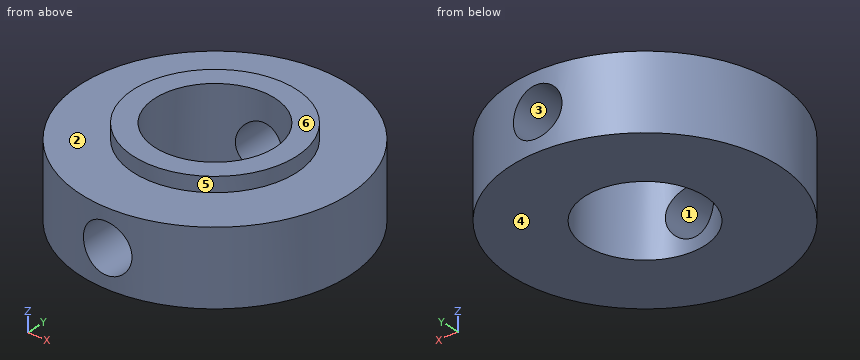
from build123d import *

# Parameters (mm, degrees)
ESQUISSE1_R                  = 9.05
ESQUISSE1_R_2                = 4.05
BOSS_EXTRU_1_DEPTH           = 5
ENL_V_MAT_EXTRU_1_DEPTH      = 14.740633173
ENL_V_MAT_EXTRU_1_DEPTH_BACK = 14.740633173
ESQUISSE2_R                  = 1.65
ESQUISSE3_R                  = 5.5
ESQUISSE3_R_2                = 4.05
BOSS_EXTRU_2_DEPTH           = 1


with BuildPart() as part:
    # Esquisse1 → Boss.-Extru.1 (new body)
    with BuildSketch(Plane.XY):
        Circle(ESQUISSE1_R)
        Circle(ESQUISSE1_R_2, mode=Mode.SUBTRACT)
    extrude(amount=BOSS_EXTRU_1_DEPTH)

    # Esquisse2 → Enlèv. mat.-Extru.1 (cut, two sides: drawn at the far end of the back side and taken through both)
    with BuildSketch(Plane(origin=(0, 0, 0), x_dir=(1, 0, 0), z_dir=(0, 1, 0)).offset(-ENL_V_MAT_EXTRU_1_DEPTH_BACK)):
        with Locations(Location((0, -2.5, 0), (0, 0, 270))):
            Circle(ESQUISSE2_R)
    extrude(amount=ENL_V_MAT_EXTRU_1_DEPTH + ENL_V_MAT_EXTRU_1_DEPTH_BACK, mode=Mode.SUBTRACT)

    # Esquisse3 → Boss.-Extru.2 (add)
    with BuildSketch(Plane.XY.offset(5)):
        Circle(ESQUISSE3_R)
        Circle(ESQUISSE3_R_2, mode=Mode.SUBTRACT)
    extrude(amount=BOSS_EXTRU_2_DEPTH)


solid = part.part
The model under review builds one solid part; all positions refer to its coordinate system, in mm. Face numbers are marked on the shaded views. A direction names the side the tool comes from. Give positions to 0.01 mm unless a question says otherwise; leave off trailing zeros. Loops run counter-clockwise (first coordinate to the right, second up) from the corner with the lowest first, then second, coordinate; pieces in that order, holes last. Notation, with made-up numbers: (74, 43.5) -> (78, 43.5) arc R28 cw to (78, 82.5) -> close; hole circle Ø10 at (-24.75, -30). An arc over 180 degrees is marked (long way). Answer as a JSON object with one key per item and string values. Group by question number.
Q1. Tool access review of the marked faces 1 and 2: name each direction out of +Z, -Z, +X, -X, +Y, -Y from which nothing blocks a thin tool from reaching the whole face with its end or side.
Q2. Take a section at B-B (x = 0). Write out the cut boundary in (y, z), plus the area to 3 significant figures.
Q3. Take a section at D-D (z = 2.5). Write out the cut boundary in (x, y).
Q4. Draft analysis for pull direction Z (two halves, no side actions). For the marked faces 3, 4, 5 and 6, state which applies: pulls with the +Z half, pulls with the -Z half, needs draft (parallel to the pull), parting line crosses it, or undercut.
Q5. Wall thickness on line 1 along Z through (x, y) = (0, -6.35); line 2 along Z through (x, y) = (-6.75, -2); line 3 along X through (y, z) = (-6.15, 2.5): over which ranges is each line inside the solid? List them lowest first.
Q6. Take a section at A-A (y = 0). Write out the cut boundary in (x, z).
Q7. Insertion check: pin 1 (1 mm diameter, centred on x = -2, z = 3.5, fed in from +Y); pin 2 (3 mm diameter, centred on x = 0, z = 2.5, fed in from -Y); pin 3 (1.5 mm diameter, centred on x = 4, z = 3.5, fed in from -Y); pin 4 (3 mm diameter, centred on x = -7, y = 2.5, fed in from +Z). Each pin has a flat end and moves straight along its axis. Give the tip position at first contact, or say it passes through.
Q8. Take a section at C-C (y = 4.5). Write out the cut boundary in (x, z), plus the area to 3 significant figures.
Answer below:
{
 "1": {"face 1": "+Y, -Y", "face 2": "+Z"},
 "2": {"outline": "(-9.05, 0) -> (-4.05, 0) -> (-4.05, 0.85) -> (-9.05, 0.85) -> close; (-9.05, 4.15) -> (-4.05, 4.15) -> (-4.05, 6) -> (-5.5, 6) -> (-5.5, 5) -> (-9.05, 5) -> close; (4.05, 0) -> (9.05, 0) -> (9.05, 0.85) -> (4.05, 0.85) -> close; (4.05, 4.15) -> (9.05, 4.15) -> (9.05, 5) -> (5.5, 5) -> (5.5, 6) -> (4.05, 6) -> close", "area": "19.9 mm2"},
 "3": {"outline": "(-1.65, -8.9) -> (-1.65, -3.7) arc R4.05 cw to (-1.65, 3.7) -> (-1.65, 8.9) arc R9.05 ccw to start; (1.65, -8.9) arc R9.05 ccw to (1.65, 8.9) -> (1.65, 3.7) arc R4.05 cw to (1.65, -3.7) -> close"},
 "4": {"face 3": "undercut", "face 4": "pulls with the -Z half", "face 5": "needs draft", "face 6": "pulls with the +Z half"},
 "5": {"line 1": "z = 0 to 0.85, 4.15 to 5", "line 2": "z = 0 to 5", "line 3": "x = -6.64 to -1.65, 1.65 to 6.64"},
 "6": {"outline": "(-9.05, 0) -> (-4.05, 0) -> (-4.05, 6) -> (-5.5, 6) -> (-5.5, 5) -> (-9.05, 5) -> close; (4.05, 0) -> (9.05, 0) -> (9.05, 5) -> (5.5, 5) -> (5.5, 6) -> (4.05, 6) -> close"},
 "7": {"pin 1": "stops at y = 8.92", "pin 2": "passes through", "pin 3": "stops at y = -8.45", "pin 4": "stops at z = 5"},
 "8": {"outline": "(-7.85, 0) -> (7.85, 0) -> (7.85, 5) -> (3.16, 5) -> (3.16, 6) -> (-3.16, 6) -> (-3.16, 5) -> (-7.85, 5) -> close; hole circle Ø3.3 at (0, 2.5)", "area": "76.3 mm2"}
}
